Autodesk Inventor part; units mm, degrees
ref_plane "YZ Plane" through (0, 0, 0) normal (1, 0, 0) x (0, 1, 0)
ref_plane "XZ Plane" through (0, 0, 0) normal (0, 1, 0) x (-1, 0, 0)
ref_plane "XY Plane" through (0, 0, 0) normal (0, 0, 1) x (1, 0, 0)
sketch "Sketch1" plane through (0, 0, 0) normal (0, 0, 1) x (1, 0, 0)
  line L0 (0, 0) -> (25.4, 0)
  line L1 (25.4, 0) -> (25.4, 25.4)
  line L2 (25.4, 25.4) -> (0, 25.4)
  line L3 (0, 25.4) -> (0, 0)
  line L4 (25.4, 25.4) -> (1.5875, 25.4)
  line L5 (1.5875, 25.4) -> (1.5875, 1.5875)
  line L6 (1.5875, 1.5875) -> (25.4, 1.5875)
  line L7 (25.4, 1.5875) -> (25.4, 25.4)
  dimension "d0" = 1.5875
  dimension "d1" = 1.5875
  dimension "d2" = 25.4
  dimension "d3" = 25.4
extrude "Extrusion1" add sketch "Sketch1" along normal blind 225.425 contours L3 L2 L5 L6 L1 L0
sketch "Sketch2" plane through (0, 0, 0) normal (0, -1, 0) x (1, 0, 0)
  line L0 (25.4, 225.425) -> (0, 225.425)
  line L1 (0, 0) -> (0, 225.425)
  line L2 (25.4, 0) -> (25.4, 225.425)
  circle A0 centre (7.9375, 219.075) radius 1.5875
  circle A1 centre (19.05, 206.375) radius 1.5875
  line L3 (0, 112.7125) -> (25.4, 112.7125)
  circle A2 centre (7.9375, 6.35) radius 1.5875
  circle A3 centre (19.05, 19.05) radius 1.5875
  dimension "d6" = 3.175
  dimension "d7" = 6.35
  dimension "d8" = 7.9375
  dimension "d9" = 19.05
  dimension "d10" = 6.35
extrude "Extrusion2" cut sketch "Sketch2" against normal blind 225.425 contours A0 | A1 | A2 | A3
sketch "Sketch3" plane through (0, 0, 0) normal (-1, 0, 0) x (0, 0, 1)
  line L0 (225.425, 0) -> (225.425, 25.4)
  line L1 (0, 25.4) -> (225.425, 25.4)
  line L2 (0, 25.4) -> (0, 0)
  line L3 (0, 0) -> (225.425, 0)
  circle A0 centre (112.7125, 15.875) radius 3.175
  line L4 (0, 1.5875) -> (100.0125, 25.4)
  line L5 (125.4125, 25.4) -> (225.425, 1.5875)
  dimension "d13" = 6.35
  dimension "d14" = 15.875
  dimension "d15" = 112.7125
  dimension "d16" = 1.5875
  dimension "d17" = 1.5875
  dimension "d18" = 12.7
  dimension "d19" = 25.4
extrude "Extrusion3" cut sketch "Sketch3" against normal blind 225.425 contours L5 L1 L0 | L2 L1 L4 | A0
equation "\"d0\" = d1"
equation "\"d3\" = d2"
equation "\"d18\" = 0.5 * d19"
properties part number "8 ball top lift point"
Build history of the part. All positions in model axes, mm. A direction names the side the tool comes from. Round coordinates to 2 decimals unless told otherwise and drop trailing zeros. Order: outer loops, then holes, each group sorted by start corner. A loop starts at its lowest first (then second) coordinate and runs counter-clockwise, first axis right, second up. Notation, with made-up numbers: (-38.5, 7) -> (1.5, 7) arc R12 ccw to (1.5, 17) -> close; hole circle Ø2 at (87.25, -4.75). An arc over 180 degrees is marked (long way). Answer in a Markdown table with one row per item.
1) Band-saw the part on B-B on x = 12.75. Give the cut face in (y, z) (1 decimal), and give its area (3 significant figures).
Values:
| item | result |
|---|---|
| outline | (0, 0) -> (1.6, 0) -> (1.6, 225.4) -> (0, 225.4) -> close |
| area | 358 mm2 |
2) Wall check: L1, parallel to Z at x = 19.05, y = 1.1 (1 decimal); L2, parallel to Y at x = 18, z = 208. Give the ranges that are in metal, low to high.
Values:
| item | result |
|---|---|
| L1 | 0 to 17.5, 20.6 to 204.8, 208 to 225.4 |
| L2 | 0 to 1.59 |
3) Band-saw the part on D-D on y = 8.25. Give the cut face in (x, z), and give its area (3 significant figures).
Values:
| item | result |
|---|---|
| outline | (0, 27.98) -> (1.59, 27.98) -> (1.59, 197.44) -> (0, 197.44) -> close |
| area | 269 mm2 |
4) Band-saw the part on A-A on z = 26. Give the cut face in (x, y), and give its area (4 significant figures).
Values:
| item | result |
|---|---|
| outline | (0, 0) -> (25.4, 0) -> (25.4, 1.59) -> (1.59, 1.59) -> (1.59, 7.78) -> (0, 7.78) -> close |
| area | 50.15 mm2 |
5) Band-saw the part on C-C on z = 165. Give the cut face in (x, y).
Values:
| item | result |
|---|---|
| outline | (0, 0) -> (25.4, 0) -> (25.4, 1.59) -> (1.59, 1.59) -> (1.59, 15.97) -> (0, 15.97) -> close |
6) Pin check, flat tips, straight feed: P1, Ø3.5, axis at x = 7.94, z = 219.08, coming from the +Y side; P2, Ø12, axis at y = 8.5, z = 112.5, coming from the +X side. Stop position of each tip, or through.
Values:
| item | result |
|---|---|
| P1 | y = 1.59 |
| P2 | x = 1.59 |
7) Mould opens along Z. For faces 3 (the flat face through (0.78, 13.33, 49.31)), 4 (the flat face through (0.78, 13.66, 174.72)), 5 (the flat face through (13, 1.588, 111)), 6 (the cylindrical face through (0.78, 16.83, 115.74)) say: released by +Z, released by -Z, zero draft, split by the parting line, or undercut.
Values:
| item | result |
|---|---|
| face 3 | released by -Z |
| face 4 | released by +Z |
| face 5 | zero draft |
| face 6 | undercut |
8) Which spindle directions (+Z, -Z, +X, -X, +Y, -Y) get a long thin tool onto all of the face, cutting with end or side? Do faces 1 (the flat face through (13, 0, 111)), 2 (the flat face through (1.588, 11, 111)). Say none if no direction does.
Values:
| item | result |
|---|---|
| face 1 | +Z, -Z, +X, -X, -Y |
| face 2 | +Z, -Z, +X, +Y |
